Source: CAD feature listing. Evaluate the final solid. Frame: model axes, mm. A direction names the side the tool comes from. Round coordinates to 2 decimals unless told otherwise and drop trailing zeros. Order: outer loops, then holes, each group sorted by start corner. A loop starts at its lowest first (then second) coordinate and runs counter-clockwise, first axis right, second up. Notation, with made-up numbers: M 72,-25 L 108,-25 A23 cw 108,-3 Z; hole C -32.75,-34 d8. An arc over 180 degrees is marked long. Answer as CSV lines item,"result". Start each with the question number.
Item 1: Section query D-D on z = -8. Return the cut outline in (x, y).
Item 2: Pull-direction query (X, two-part tool) for faces 1 (the face through (-30, 1, -27)), 2 (the face through (-1, 0, 20)), 3 (the face through (-48.859, 1.014, -28.797)); classes: +X half, -X half, draft (parallel to the pull), parting line (faces both ways), or undercut.
Item 3: Section query A-A on x = -45. Return the cut outline in (y, z), plus the area to 3 significant figures.
Item 4: Section query C-C on x = 25. Return the cut outline in (y, z), plus the area to 3 significant figures.
Item 5: Set-up query: faces 4 (the face through (-44, 1, 30)), 5 (the face through (0, 1, 15)), 6 (the face through (-30, 1, 27)). Return all of +Z, -Z, +X, -X, +Y, -Y with unobstructed straight access to the full face (end or side cutting, diameter ignored); none if empty.
Item 6: First-contact query: P1, Ø5, axis at x = 15, z = 25, coming from the -Y side; P2, Ø2.5, axis at x = 16, z = 20, coming from the -Y side; P3, Ø0.8, axis at y = 1.5, z = -28.5, coming from the +X side; P4, Ø1.1, axis at y = 0.5, z = 28.5, coming from the -X side. Flat tips, straight axial feed; report the tip coordinate or a pass-through.
Item 7: Line query: line 1 (X direction, y = 0.8, z = 25); line 2 (Z direction, x = 5, y = 0.85); line 3 (X direction, y = 0.9, z = -5.5). Output: solid intervals per line, ascending. Write a range as [from, to].
Item 8: Section query B-B on z = -25. Return the cut outline in (x, y), plus the area to 3 significant figures.
from build123d import *

# Parameters (mm, degrees)
SKETCH_1_W           = 100
SKETCH_1_H           = 60
EXTRUDE_1_DEPTH      = 2
SKETCH_4_W           = 40
SKETCH_4_H           = 30
CUT_EXTRUDE_3_DEPTH  = 59.343808583
SKETCH_6_R           = 1.5
CUT_EXTRUDE_5_DEPTH  = 59.343808583
SKETCH_7_W           = 20
SKETCH_7_H           = 3
CUT_EXTRUDE_6_DEPTH  = 59.343808583
FILLET_1_R           = 4
FILLET_2_R           = 1
SKETCH_8_R           = 1.5
CUT_EXTRUDE_7_DEPTH  = 59.343808583
SKETCH_9_W           = 4
SKETCH_9_H           = 40
CUT_EXTRUDE_9_DEPTH  = 59.343808583
FILLET_START         = -1
FILLET_3_DEPTH       = 4
FILLET_3_2_DEPTH     = 2
SKETCH_10_R          = 1.5
CUT_EXTRUDE_10_DEPTH = 59.343808583


with BuildPart() as part:
    # 草图1 → 凸台-拉伸1 (new body)
    with BuildSketch(Plane(origin=(0, 0, 0), x_dir=(1, 0, 0), z_dir=(0, 1, 0))):
        Rectangle(SKETCH_1_W, SKETCH_1_H)
    extrude(amount=EXTRUDE_1_DEPTH)

    # 草图4 → 切除-拉伸3 (cut, through all)
    with BuildSketch(Plane(origin=(0, 2, 0), x_dir=(1, 0, 0), z_dir=(0, 1, 0))):
        Rectangle(SKETCH_4_W, SKETCH_4_H)
    extrude(amount=-CUT_EXTRUDE_3_DEPTH, mode=Mode.SUBTRACT)

    # 草图6 → 切除-拉伸5 (cut, through all)
    with BuildSketch(Plane(origin=(0, 2, 0), x_dir=(1, 0, 0), z_dir=(0, 1, 0))):
        with Locations(Location((-45, 25, 0), (0, 0, 270))):
            Circle(SKETCH_6_R)
        with Locations(Location((-45, -25, 0), (0, 0, 90))):
            Circle(SKETCH_6_R)
        with Locations(Location((45, -25, 0), (0, 0, 270))):
            Circle(SKETCH_6_R)
        with Locations(Location((45, 25, 0), (0, 0, 90))):
            Circle(SKETCH_6_R)
    extrude(amount=-CUT_EXTRUDE_5_DEPTH, mode=Mode.SUBTRACT)

    # 草图7 → 切除-拉伸6 (cut, through all)
    with BuildSketch(Plane(origin=(0, 2, 0), x_dir=(1, 0, 0), z_dir=(0, 1, 0))):
        with Locations((-30, 28.5)):
            Rectangle(SKETCH_7_W, SKETCH_7_H)
        with Locations((-30, -28.5)):
            Rectangle(SKETCH_7_W, SKETCH_7_H)
        with Locations((30, -28.5)):
            Rectangle(SKETCH_7_W, SKETCH_7_H)
        with Locations((30, 28.5)):
            Rectangle(SKETCH_7_W, SKETCH_7_H)
    extrude(amount=-CUT_EXTRUDE_6_DEPTH, mode=Mode.SUBTRACT)

    # 圆角1
    fillet_1_edges = [part.edges().sort_by_distance(p)[0] for p in [
        (20, 1, -15),
        (20, 1, 15),
        (-20, 1, 15),
        (-20, 1, -15),
        (50, 1, 30),
        (-50, 1, 30),
        (-50, 1, -30),
        (50, 1, -30),
    ]]
    fillet(fillet_1_edges, radius=FILLET_1_R)

    # 圆角2
    fillet_2_edges = [part.edges().sort_by_distance(p)[0] for p in [
        (40, 1, -30),
        (40, 1, -27),
        (20, 1, -27),
        (20, 1, -30),
        (40, 1, 30),
        (20, 1, 30),
        (20, 1, 27),
        (40, 1, 27),
        (-40, 1, 30),
        (-40, 1, 27),
        (-20, 1, 27),
        (-20, 1, 30),
        (-40, 1, -27),
        (-40, 1, -30),
        (-20, 1, -30),
        (-20, 1, -27),
    ]]
    fillet(fillet_2_edges, radius=FILLET_2_R)

    # 草图8 → 切除-拉伸7 (cut, through all)
    with BuildSketch(Plane(origin=(0, 2, 0), x_dir=(1, 0, 0), z_dir=(0, 1, 0))):
        with Locations(Location((-15, 25, 0), (0, 0, 270))):
            Circle(SKETCH_8_R)
        with Locations(Location((-15, -25, 0), (0, 0, 90))):
            Circle(SKETCH_8_R)
        with Locations(Location((15, -25, 0), (0, 0, 270))):
            Circle(SKETCH_8_R)
        with Locations(Location((15, 25, 0), (0, 0, 90))):
            Circle(SKETCH_8_R)
    extrude(amount=-CUT_EXTRUDE_7_DEPTH, mode=Mode.SUBTRACT)

    # 草图9 → 切除-拉伸9 (cut, through all)
    with BuildSketch(Plane(origin=(0, 2, 0), x_dir=(1, 0, 0), z_dir=(0, 1, 0))):
        with Locations((-48, 0)):
            Rectangle(SKETCH_9_W, SKETCH_9_H)
        with Locations((48, 0)):
            Rectangle(SKETCH_9_W, SKETCH_9_H)
    extrude(amount=-CUT_EXTRUDE_9_DEPTH, mode=Mode.SUBTRACT)

    # 圆角3: read off the stored shape, not the designer's step
    # 圆角3 outline → 圆角3 (cut)
    with BuildSketch(Plane(origin=(0, 0, 0), x_dir=(1, 0, 0), z_dir=(0, 1, 0)).offset(FILLET_START)):
        with BuildLine():
            Line((50, -20), (48, -20))
            ThreePointArc((48, -20), (49.414213562, -20.585786438), (50, -22))
            Line((50, -22), (50, -20))
        make_face()
        with BuildLine():
            ThreePointArc((50, 22), (49.414213562, 20.585786438), (48, 20))
            Line((48, 20), (50, 20))
            Line((50, 20), (50, 22))
        make_face()
        with BuildLine():
            Line((-50, 20), (-48, 20))
            ThreePointArc((-48, 20), (-49.414213562, 20.585786438), (-50, 22))
            Line((-50, 22), (-50, 20))
        make_face()
        with BuildLine():
            ThreePointArc((-50, -22), (-49.414213562, -20.585786438), (-48, -20))
            Line((-48, -20), (-50, -20))
            Line((-50, -20), (-50, -22))
        make_face()
    extrude(amount=FILLET_3_DEPTH, mode=Mode.SUBTRACT)

    # Fillet 3 2 outline → Fillet 3 2 (add)
    with BuildSketch(Plane(origin=(0, 0, 0), x_dir=(1, 0, 0), z_dir=(0, 1, 0))):
        with BuildLine():
            Line((46, -20), (48, -20))
            ThreePointArc((48, -20), (46.585786438, -19.414213562), (46, -18))
            Line((46, -18), (46, -20))
        make_face()
        with BuildLine():
            Line((46, 20), (46, 18))
            ThreePointArc((46, 18), (46.585786438, 19.414213562), (48, 20))
            Line((48, 20), (46, 20))
        make_face()
        with BuildLine():
            ThreePointArc((-48, 20), (-46.585786438, 19.414213562), (-46, 18))
            Line((-46, 18), (-46, 20))
            Line((-46, 20), (-48, 20))
        make_face()
        with BuildLine():
            ThreePointArc((-46, -18), (-46.585786438, -19.414213562), (-48, -20))
            Line((-48, -20), (-46, -20))
            Line((-46, -20), (-46, -18))
        make_face()
    extrude(amount=FILLET_3_2_DEPTH)

    # 草图10 → 切除-拉伸10 (cut, through all)
    with BuildSketch(Plane(origin=(0, 2, 0), x_dir=(1, 0, 0), z_dir=(0, 1, 0))):
        with Locations(Location((-25, 0, 0), (0, 0, 270))):
            Circle(SKETCH_10_R)
        with Locations(Location((-16, 20, 0), (0, 0, 270))):
            Circle(SKETCH_10_R)
        with Locations(Location((-16, -20, 0), (0, 0, 90))):
            Circle(SKETCH_10_R)
        with Locations(Location((16, 20, 0), (0, 0, 90))):
            Circle(SKETCH_10_R)
        with Locations(Location((16, -20, 0), (0, 0, 270))):
            Circle(SKETCH_10_R)
        with Locations(Location((25, 0, 0), (0, 0, 90))):
            Circle(SKETCH_10_R)
        with Locations(Location((-35, 15, 0), (0, 0, 270))):
            Circle(SKETCH_10_R)
        with Locations(Location((-35, -15, 0), (0, 0, 90))):
            Circle(SKETCH_10_R)
        with Locations(Location((35, -15, 0), (0, 0, 270))):
            Circle(SKETCH_10_R)
        with Locations(Location((35, 15, 0), (0, 0, 90))):
            Circle(SKETCH_10_R)
    extrude(amount=-CUT_EXTRUDE_10_DEPTH, mode=Mode.SUBTRACT)


solid = part.part
Results:
1,outline,"M -46,0 L -20,0 L -20,2 L -46,2 Z; M 20,0 L 46,0 L 46,2 L 20,2 Z"
2,face 1,"undercut"
2,face 2,"draft"
2,face 3,"-X half"
3,outline,"M 0,-30 L 2,-30 L 2,-26.5 L 0,-26.5 Z; M 0,-23.5 L 2,-23.5 L 2,23.5 L 0,23.5 Z; M 0,26.5 L 2,26.5 L 2,30 L 0,30 Z"
3,area,"108 mm^2"
4,outline,"M 0,-27 L 2,-27 L 2,-1.5 L 0,-1.5 Z; M 0,1.5 L 2,1.5 L 2,27 L 0,27 Z"
4,area,"102 mm^2"
5,face 4,"+Z, +X, -X, +Y, -Y"
5,face 5,"+Y, -Y"
5,face 6,"+Z, +Y, -Y"
6,P1,"y = 0"
6,P2,"through"
6,P3,"x = 49.4"
6,P4,"x = -49.49"
7,line 1,"[-50, -46.5], [-43.5, -16.5], [-13.5, 13.5], [16.5, 43.5], [46.5, 50]"
7,line 2,"[-30, -15], [15, 30]"
7,line 3,"[-46, -20], [20, 46]"
8,outline,"M -50,0 L -46.5,0 L -46.5,2 L -50,2 Z; M -43.5,0 L -16.5,0 L -16.5,2 L -43.5,2 Z; M -13.5,0 L 13.5,0 L 13.5,2 L -13.5,2 Z; M 16.5,0 L 43.5,0 L 43.5,2 L 16.5,2 Z; M 46.5,0 L 50,0 L 50,2 L 46.5,2 Z"
8,area,"176 mm^2"
